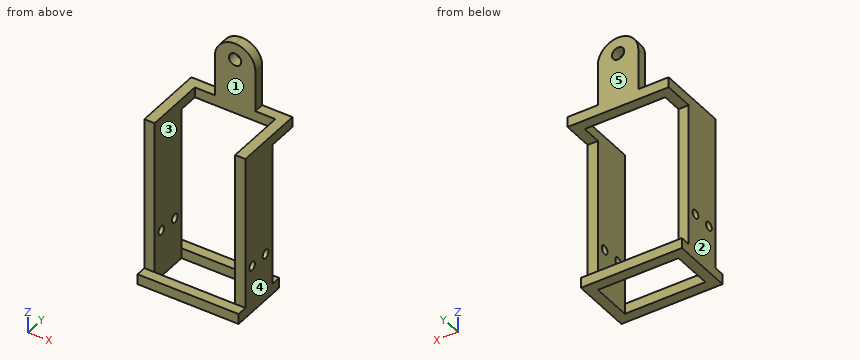
Autodesk Inventor part; units mm, degrees
ref_plane "YZ Plane" through (0, 0, 0) normal (1, 0, 0) x (0, 1, 0)
ref_plane "XZ Plane" through (0, 0, 0) normal (0, 1, 0) x (-1, 0, 0)
ref_plane "XY Plane" through (0, 0, 0) normal (0, 0, 1) x (1, 0, 0)
sketch "Sketch1" plane through (0, 0, 0) normal (0, 0, 1) x (1, 0, 0)
  line L0 (-19.603, -9.85) -> (19.603, -9.85)
  line L1 (19.603, -9.85) -> (19.603, 9.85)
  line L2 (19.603, 9.85) -> (-19.603, 9.85)
  line L3 (-19.603, 9.85) -> (-19.603, -9.85)
  line L4 (-19.603, -9.85) -> (19.603, 9.85) construction
  line L5 (19.603, -9.85) -> (-19.603, 9.85) construction
  line L6 (-24.603, 14.85) -> (24.603, 14.85)
  line L7 (24.603, 14.85) -> (24.603, -14.85)
  line L8 (24.603, -14.85) -> (-24.603, -14.85)
  line L9 (-24.603, -14.85) -> (-24.603, 14.85)
  point P0 (0, 0)
  dimension "d0" = 39.206
  dimension "d1" = 19.7
  dimension "d2" = 5
extrude "Extrusion1" add sketch "Sketch1" along normal blind 5
sketch "Sketch2" plane through (0, 0, 5) normal (0, 0, 1) x (1, 0, 0)
  line L0 (-24.603, 14.85) -> (-24.603, -14.85) construction
  line L1 (-24.603, 14.85) -> (-24.603, -14.85) construction
  line L2 (24.603, 14.85) -> (-24.603, 14.85) construction
  line L3 (-24.603, 14.85) -> (24.603, 14.85) construction
  line L4 (24.603, -14.85) -> (24.603, 14.85) construction
  line L5 (24.603, 14.85) -> (24.603, -14.85) construction
  line L6 (24.603, -14.85) -> (-24.603, -14.85) construction
  line L7 (-19.603, -9.85) -> (-19.603, 9.85)
  line L8 (-19.603, 9.85) -> (-24.603, 9.85)
  line L9 (-24.603, 9.85) -> (-24.603, -9.85)
  line L10 (-24.603, -9.85) -> (-19.603, -9.85)
  line L11 (-19.603, -9.85) -> (-19.603, 9.85)
  line L12 (19.603, 9.85) -> (19.603, -9.85)
  line L13 (19.603, 9.85) -> (24.603, 9.85)
  line L14 (24.603, 9.85) -> (24.603, -9.85)
  line L15 (24.603, -9.85) -> (19.603, -9.85)
  line L16 (19.603, -9.85) -> (19.603, 9.85)
  point P0 (0, 0)
extrude "Extrusion2" add sketch "Sketch2" along normal blind 75
sketch "Sketch3" plane through (0, 0, 0) normal (1, 0, 0) x (0, 1, 0)
  circle A0 centre (4.925, 23.111) radius 2.1
  line L0 (14.85, 0) -> (14.85, 5)
  line L1 (14.85, 5) -> (9.85, 5)
  circle A1 centre (-4.925, 23.111) radius 2.1
  line L2 (-14.85, 0) -> (-14.85, 5)
  line L3 (-9.85, 5) -> (-14.85, 5)
  point P0 (0, 0)
  point P1 (-12.35, 5)
  dimension "d7" = 4.2
  dimension "d8" = 9.925
  dimension "d9" = 18.111
  dimension "d10" = 4.2
  dimension "d11" = 9.925
  dimension "d12" = 18.111
extrude "Extrusion3" cut sketch "Sketch3" along normal through all both and the other way through all
sketch "Sketch4" plane through (0, 0, 0) normal (1, 0, 0) x (0, 1, 0)
  line L0 (-9.85, 80) -> (9.85, 80) construction
  line L1 (0, 80) -> (0, 0) construction
  line L2 (24.603, 80) -> (19.603, 80)
  line L3 (19.603, 80) -> (19.603, 75)
  line L4 (19.603, 75) -> (24.603, 75)
  line L5 (24.603, 75) -> (24.603, 80)
  line L6 (14.85, 0) -> (-14.85, 0)
  point P0 (19.603, 77.5)
  dimension "d29" = 5
  dimension "d30" = 5
  dimension "d31" = 19.603
  dimension "d32" = 75
extrude "Extrusion4" add sketch "Sketch4" along normal mid plane 49.206
sketch "Sketch5" plane through (0, 0, 80) normal (0, 0, 1) x (1, 0, 0)
  line L0 (-24.603, -9.85) -> (-24.603, 14.85)
  line L1 (24.603, -9.85) -> (24.603, 14.85)
  line L2 (-24.603, 24.603) -> (24.603, 24.603)
  line L3 (-9.85, 24.603) -> (9.85, 24.603)
  line L4 (9.85, 24.603) -> (9.85, 19.603)
  line L5 (9.85, 19.603) -> (-9.85, 19.603)
  line L6 (-9.85, 19.603) -> (-9.85, 24.603)
  line L7 (24.603, 24.603) -> (24.603, 19.603)
  line L8 (-24.603, 19.603) -> (-24.603, 24.603)
  point P0 (0, 0)
  point P1 (9.85, 22.103)
  point P2 (-24.603, 22.103)
  point P3 (9.85, 24.603)
  dimension "d33" = 19.7
  dimension "d34" = 5
  dimension "d35" = 14.753
  dimension "d36" = 14.753
extrude "Extrusion5" add sketch "Sketch5" along normal blind 30
sketch "Sketch7" plane through (19.603, 9.85, 5) normal (0, 1, 0) x (1, 0, 0)
  line L0 (-39.206, 0) -> (-39.206, -75)
  line L1 (-39.206, -75) -> (-44.206, -75)
  line L2 (-44.206, -75) -> (-44.206, -70)
  line L3 (-44.206, -70) -> (-39.206, -70)
  line L4 (-39.206, -70) -> (-39.206, -75)
  line L5 (0, 0) -> (0, -75)
  line L6 (0, -75) -> (5, -75)
  line L7 (5, -75) -> (5, -70)
  line L8 (5, -70) -> (0, -70)
  line L9 (0, -70) -> (0, -75)
  point P0 (-19.603, 5)
  point P1 (-39.206, -70)
  point P2 (0, -70)
  dimension "d37" = 5
  dimension "d38" = 5
  dimension "d39" = 5
  dimension "d40" = 5
extrude "Extrusion7" add sketch "Sketch7" along normal through all
sketch "Sketch8" plane through (-24.603, 24.603, 75) normal (0, 1, 0) x (1, 0, 0)
  line L0 (14.753, -35) -> (34.453, -35) construction
  line L1 (24.603, -35) -> (24.603, 0) construction
  line L2 (5, 0) -> (44.206, 0) construction
  circle A0 centre (24.603, -27) radius 3
  point P0 (24.603, 75)
  point P1 (0, 0)
  point P2 (49.206, 0)
  dimension "d43" = 6
  dimension "d44" = 8
extrude "Extrusion8" cut sketch "Sketch8" against normal through all
fillet "Fillet1" radius 9.85 2 edges at (9.85, 22.103, 110) (-9.85, 22.103, 110)
properties part number "Part2_cage"
The listing builds one solid part. Answer for the finished solid, in the listing's coordinates (mm). Face numbers are marked on the shaded views. A direction names the side the tool comes from. Coordinates: 2 decimals unless noted, no trailing zeros. Write each loop counter-clockwise with the first axis right and the second up, starting at its lowest first coordinate (ties: lowest second). Pieces come first, ordered by that corner, then holes. Notation, with made-up numbers: (-36, 24.5) - (-20, 24.5) arc R4 cw to (-20, 31.5) - close; hole circle Ø8 at (24, 41.5). An arc over 180 degrees is marked (long way). Put each result on its own line as item: value.
1. Flat-ended cylindrical pins translate along their axes: pin 1 Ø5.5 at (y, z) = (4.925, 23.111) entering from -X; pin 2 Ø4 at (y, z) = (22.5, 95) entering from -X; pin 3 Ø2.5 at (x, z) = (-23, 56.5) entering from -Y; pin 4 Ø2.5 at (x, z) = (1, 2.5) entering from +Y. Find the tip coordinate at first contact, or state that the pin passes through.
Answer sheet:
pin 1: stops at x = -24.6
pin 2: stops at x = -9.85
pin 3: stops at y = -9.85
pin 4: stops at y = 14.85
2. The part is cut by section B-B on z = 31. Give the vertices of the cut face in (x, y), plus the area to 3 significant figures.
Answer sheet:
outline: (-24.6, -9.85) - (-19.6, -9.85) - (-19.6, 9.85) - (-24.6, 9.85) - close; (19.6, -9.85) - (24.6, -9.85) - (24.6, 9.85) - (19.6, 9.85) - close
area: 197 mm^2
3. The part is cut by section C-C on z = 102. Give the vertices of the cut face in (x, y).
Answer sheet:
outline: (-9.67, 19.6) - (-3, 19.6) - (-3, 24.6) - (-9.67, 24.6) - close; (3, 19.6) - (9.67, 19.6) - (9.67, 24.6) - (3, 24.6) - close
4. The part is cut by section A-A on x = -17.5. Give the vertices of the cut face in (y, z), plus the area to 3 significant figures.
Answer sheet:
outline: (-14.85, 0) - (-9.85, 0) - (-9.85, 5) - (-14.85, 5) - close; (9.85, 0) - (14.85, 0) - (14.85, 5) - (9.85, 5) - close; (19.6, 75) - (24.6, 75) - (24.6, 80) - (19.6, 80) - close
area: 75.0 mm^2
5. The part is cut by section D-D on z = 87.5. Give the vertices of the cut face in (x, y).
Answer sheet:
outline: (-9.85, 19.6) - (9.85, 19.6) - (9.85, 24.6) - (-9.85, 24.6) - close
6. Determine the mould class of the marked faces 3, 4 and 5 for opening direction X: pulls with the +X half, pulls with the -X half, needs draft (parallel to the pull), parting line crosses it, or undercut.
Answer sheet:
face 3: undercut
face 4: pulls with the +X half
face 5: needs draft
7. Find the intervals of material crossed by line 1 along X through (y, z) = (-9, 54); line 2 along Y through (x, z) = (-1, 90.5); line 3 along Z through (x, y) = (11.5, 11), in increasing order. Write a range as from..to.
Answer sheet:
line 1: x = -24.6..-19.6, 19.6..24.6
line 2: y = 19.6..24.6
line 3: z = 0..5
8. A tool of negligible diameter and unlimited length cuts with its end or side. For the marked faces 1 and 2, from which of +Z, -Z, +X, -X, +Y, -Y can it reach the whole face along a straight path? Write none if from no direction.
Answer sheet:
face 1: +Z, -Z, -Y
face 2: +Z, -Z, -X, +Y, -Y
